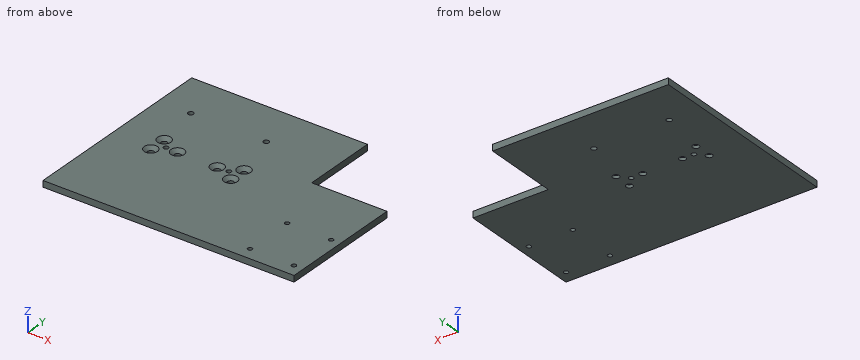
from build123d import *

# Parameters (mm, degrees)
F0_W           = 127
F0_H           = 3.175
F1_DEPTH       = 50.8
F3_D           = 3.3
F3_CSINK_D     = 6.72
F3_CSINK_ANGLE = 90
F5_D           = 2.4
F6_W           = 38.1
F6_H           = 38.1
F7_DEPTH       = 3.176
F9_D           = 2.2606
F11_D          = 2.7051


with BuildPart() as f1:
    # F0 (on Front) → F1 (new body, symmetric)
    with BuildSketch(Plane.XZ):
        with Locations((-63.5, 1.5875)):
            Rectangle(F0_W, F0_H)
    extrude(amount=F1_DEPTH, both=True)

    # F3 (through all)
    with Locations(Plane.XY.offset(3.175)):
        with Locations((-66.294, 4.572), (-66.294, -4.572), (-76.454, 0), (-96.52, 0), (-106.68, 4.572), (-106.68, -4.572)):
            CounterSinkHole(F3_D / 2, F3_CSINK_D / 2, counter_sink_angle=F3_CSINK_ANGLE)

    # F5 (through all)
    with Locations(Plane.XY.offset(3.175)):
        with Locations((-102.362, 0), (-70.612, 0)):
            Hole(F5_D / 2)

    # F6 (on face) → F7 (cut, through all)
    with BuildSketch(Plane.XY.offset(3.175)):
        with Locations((-19.05, 31.75)):
            Rectangle(F6_W, F6_H)
    extrude(amount=-F7_DEPTH, mode=Mode.SUBTRACT)

    # F9 (through all)
    with Locations(Plane.XY.offset(3.175)):
        with Locations((-26.9875, -44.45), (-26.9875, -19.05), (-4.7625, -19.05), (-4.7625, -44.45)):
            Hole(F9_D / 2)

    # F11 (through all)
    with Locations(Plane.XY.offset(3.175)):
        with Locations((-110.49, 27.94), (-72.39, 27.94)):
            Hole(F11_D / 2)


solid = f1.part
Read the model definition and answer for the solid it produces. Units are mm, in the model's axes. Round coordinates to 2 decimals unless told otherwise and drop trailing zeros. Write each loop counter-clockwise with the first axis right and the second up, starting at its lowest first coordinate (ties: lowest second). Pieces come first, ordered by that corner, then holes.
1. The part is cut by section C-C, the plane z = 2.5. State how many separate pieces and enclosed holes the cut face has, then the cut area to 3 significant figures.
2. Given pin 1 Ø10 at (x, y) = (-101, -27) entering from -Z; pin 2 Ø1 at (x, z) = (-19, 1.5) entering from +Y; pin 3 Ø5.5 at (x, y) = (-66.294, -4.572) entering from +Z (3 decimals); pin 4 Ø1 at (y, z) = (25, 2) entering from +X, each flat-ended and moving along its own axis, determine where each tip first touches the part or whether it passes through.
3. The part is cut by section A-A, the plane y = 27.94. Determine the outline of the cut face in (x, z) (3 decimals), then the cut area to 3 significant figures.
4. Straight lines are drawn through the part: L1, parallel to Y at x = -106.68, z = 1.1; L2, parallel to Y at x = -105.5, z = 0.3; L3, parallel to X at y = -44, z = 1.35. For each, find the intervals that lie inside material, in ascending order.
5. The part is cut by section D-D, the plane x = -17.5. Determine the outline of the cut face in (y, z) (3 decimals).
6. The part is cut by section B-B, the plane x = -106.68. Determine the outline of the cut face in (y, z) (3 decimals).
Values:
1. separate pieces: 1
1. enclosed holes: 14
1. area: 11,300 mm2
2. pin 1: stops at z = 0
2. pin 2: stops at y = 12.7
2. pin 3: stops at z = 2.565
2. pin 4: stops at x = -38.1
3. outline: (-127, 0) - (-111.843, 0) - (-111.843, 3.175) - (-127, 3.175) - close; (-109.137, 0) - (-73.743, 0) - (-73.743, 3.175) - (-109.137, 3.175) - close; (-71.037, 0) - (-38.1, 0) - (-38.1, 3.175) - (-71.037, 3.175) - close
3. area: 265 mm2
4. L1: y = -50.8 to -6.22, -2.92 to 2.92, 6.22 to 50.8
4. L2: y = -50.8 to -5.73, -3.42 to 3.42, 5.73 to 50.8
4. L3: x = -127 to -28.02, -25.95 to -5.8, -3.73 to 0
5. outline: (-50.8, 0) - (12.7, 0) - (12.7, 3.175) - (-50.8, 3.175) - close
6. outline: (-50.8, 0) - (-6.222, 0) - (-6.222, 1.465) - (-7.932, 3.175) - (-50.8, 3.175) - close; (-2.922, 0) - (2.922, 0) - (2.922, 1.465) - (1.212, 3.175) - (-1.212, 3.175) - (-2.922, 1.465) - close; (6.222, 0) - (50.8, 0) - (50.8, 3.175) - (7.932, 3.175) - (6.222, 1.465) - close
